Design review of the part built by this model. Coordinates are the model's own, in mm. Round coordinates to 2 decimals unless told otherwise and drop trailing zeros. Write each loop counter-clockwise with the first axis right and the second up, starting at its lowest first coordinate (ties: lowest second). Pieces come first, ordered by that corner, then holes. Notation, with made-up numbers: (-17.5, 80.5) -> (36.5, 80.5) arc R14 ccw to (36.5, 92.5) -> close; hole circle Ø5 at (56, -18.75). An arc over 180 degrees is marked (long way). One line per question, with ' | ' between items. Start each with the question number.
1) For probe 1 along Y at (x, z) = (0, 180.5); probe 2 along Y at (x, z) = (-195.5, -178.5); probe 3 along Z at (x, y) = (-315, -523.5), list the stretches that pass through material, from the lowest coordinate up.
2) Insertion check: pin 1 Ø1.2 at (x, z) = (-552, 936) entering from -Y; pin 2 Ø0.8 at (x, z) = (635, 935.5) entering from +Y; pin 3 Ø0.5 at (y, z) = (11.5, 935.5) entering from -X. Each pin has a flat end and moves straight along its axis. Give the tip position at first contact, or say it passes through.
3) Consider section A-A (z = 16). Give the boundary of the cut face in (x, y), then the cut area to 3 significant figures.
4) Consider section B-B (z = 795.5). Give the boundary of the cut face in (x, y).
```python
from build123d import *

# Parameters (mm, degrees)
SKETCH1_R           = 100
SKETCH1_R_2         = 45
BOSS_EXTRUDE1_DEPTH = 200
FILLET1_R           = 8
FILLET2_R           = 20
CUT_EXTRUDE1_DEPTH  = 200
SKETCH3_W           = 21.544123994
SKETCH3_H           = 11.057339859
BOSS_EXTRUDE2_DEPTH = 3
FILLET3_R           = 1.5
SKETCH4_R           = 1.289060933
SKETCH4_W           = 15.13149362
SKETCH4_H           = 3.065252971
SKETCH4_W_2         = 2.299952362
SKETCH4_H_2         = 2.429436964
SKETCH4_W_3         = 1.819095979
SKETCH4_H_3         = 1.788232519
SKETCH4_W_4         = 1.827971019
SKETCH4_W_5         = 1.693323788
SKETCH4_W_6         = 1.708755518
SKETCH4_W_7         = 1.86770952
SKETCH4_W_8         = 4.247138883
SKETCH4_W_9         = 4.75974501
SKETCH4_H_4         = 1.629278517
BOSS_EXTRUDE3_DEPTH = 0.2
SKETCH5_R           = 100
BOSS_EXTRUDE4_DEPTH = 8
SCALE1_SCALE        = 15.6
SCALE2_SCALE        = 0.5


with BuildPart() as part:
    # Sketch1 → Boss-Extrude1 (new body)
    with BuildSketch(Plane.XY):
        Circle(SKETCH1_R)
        Circle(SKETCH1_R_2, mode=Mode.SUBTRACT)
    extrude(amount=BOSS_EXTRUDE1_DEPTH)

    # Fillet1
    fillet1_edges = [part.edges().sort_by_distance(p)[0] for p in [
        (-100, 0, 200),
    ]]
    fillet(fillet1_edges, radius=FILLET1_R)

    # Fillet2
    fillet2_edges = [part.edges().sort_by_distance(p)[0] for p in [
        (-45, 0, 200),
    ]]
    fillet(fillet2_edges, radius=FILLET2_R)

    # Sketch2 → Cut-Extrude1 (cut)
    with BuildSketch(Plane(origin=(0, 0, 0), x_dir=(-1, 0, 0), z_dir=(0, 0, -1))):
        with BuildLine():
            Line((-28.43159427, -34.880430721), (28.43159427, -34.880430721))
            Line((28.43159427, -34.880430721), (28.43159427, -39.361060603))
            Line((28.43159427, -39.361060603), (11.44568617, -39.361060603))
            Line((11.44568617, -39.361060603), (11.44568617, -48.0006973))
            ThreePointArc((11.44568617, -48.0006973), (0, -49.480629882), (-11.44568617, -48.0006973))
            Line((-11.44568617, -48.0006973), (-11.44568617, -39.361060603))
            Line((-11.44568617, -39.361060603), (-28.43159427, -39.361060603))
            Line((-28.43159427, -39.361060603), (-28.43159427, -34.880430721))
        make_face()
    extrude(amount=-CUT_EXTRUDE1_DEPTH, mode=Mode.SUBTRACT)

    # Sketch3 → Boss-Extrude2 (add)
    with BuildSketch(Plane.XY.offset(200)):
        with Locations((78.121999913, 5.52866993)):
            Rectangle(SKETCH3_W, SKETCH3_H)
        with Locations((-78.121999913, 5.52866993)):
            Rectangle(SKETCH3_W, SKETCH3_H)
    extrude(amount=BOSS_EXTRUDE2_DEPTH)

    # Fillet3
    fillet3_edges = [part.edges().sort_by_distance(p)[0] for p in [
        (67.349937916, 11.057339859, 201.5),
        (67.349937916, 0, 201.5),
        (88.89406191, 0, 201.5),
        (88.89406191, 11.057339859, 201.5),
        (-88.89406191, 0, 201.5),
        (-67.349937916, 0, 201.5),
        (-67.349937916, 11.057339859, 201.5),
        (-88.89406191, 11.057339859, 201.5),
    ]]
    fillet(fillet3_edges, radius=FILLET3_R)

    # Sketch4 → Boss-Extrude3 (add)
    with BuildSketch(Plane.XY.offset(203)):
        with Locations((85.270492468, 1.703597588)):
            Circle(SKETCH4_R)
        with Locations((-85.270492468, 1.703597588)):
            Circle(SKETCH4_R)
        with Locations((76.415684726, 8.024713374)):
            Rectangle(SKETCH4_W, SKETCH4_H)
        with Locations((86.244085729, 8.342621377)):
            Rectangle(SKETCH4_W_2, SKETCH4_H_2)
        with Locations((69.759485906, 4.564769617)):
            Rectangle(SKETCH4_W_3, SKETCH4_H_3)
        with Locations((72.695697416, 4.564769617)):
            Rectangle(SKETCH4_W_4, SKETCH4_H_3)
        with Locations((75.569022832, 4.564769617)):
            Rectangle(SKETCH4_W_5, SKETCH4_H_3)
        with Locations((78.358433726, 4.564769617)):
            Rectangle(SKETCH4_W_6, SKETCH4_H_3)
        with Locations((81.259344257, 4.564769617)):
            Rectangle(SKETCH4_W_7, SKETCH4_H_3)
        with Locations((85.270492469, 4.564769617)):
            Rectangle(SKETCH4_W_8, SKETCH4_H_3)
        with Locations((71.229810421, 1.703597588)):
            Rectangle(SKETCH4_W_9, SKETCH4_H_4)
        with Locations((75.569022832, 1.703597588)):
            Rectangle(SKETCH4_W_5, SKETCH4_H_4)
        with Locations((78.358433726, 1.703597588)):
            Rectangle(SKETCH4_W_6, SKETCH4_H_4)
        with Locations((81.259344257, 1.703597588)):
            Rectangle(SKETCH4_W_7, SKETCH4_H_4)
        with Locations((-81.259344257, 1.703597588)):
            Rectangle(SKETCH4_W_7, SKETCH4_H_4)
        with Locations((-78.358433726, 1.703597588)):
            Rectangle(SKETCH4_W_6, SKETCH4_H_4)
        with Locations((-75.569022832, 1.703597588)):
            Rectangle(SKETCH4_W_5, SKETCH4_H_4)
        with Locations((-71.229810421, 1.703597588)):
            Rectangle(SKETCH4_W_9, SKETCH4_H_4)
        with Locations((-85.270492469, 4.564769617)):
            Rectangle(SKETCH4_W_8, SKETCH4_H_3)
        with Locations((-81.259344257, 4.564769617)):
            Rectangle(SKETCH4_W_7, SKETCH4_H_3)
        with Locations((-78.358433726, 4.564769617)):
            Rectangle(SKETCH4_W_6, SKETCH4_H_3)
        with Locations((-75.569022832, 4.564769617)):
            Rectangle(SKETCH4_W_5, SKETCH4_H_3)
        with Locations((-72.695697416, 4.564769617)):
            Rectangle(SKETCH4_W_4, SKETCH4_H_3)
        with Locations((-69.759485906, 4.564769617)):
            Rectangle(SKETCH4_W_3, SKETCH4_H_3)
        with Locations((-86.244085729, 8.342621377)):
            Rectangle(SKETCH4_W_2, SKETCH4_H_2)
        with Locations((-76.415684726, 8.024713374)):
            Rectangle(SKETCH4_W, SKETCH4_H)
    extrude(amount=BOSS_EXTRUDE3_DEPTH)

    # Sketch5 → Boss-Extrude4 (add)
    with BuildSketch(Plane(origin=(0, 0, 0), x_dir=(-1, 0, 0), z_dir=(0, 0, -1))):
        Circle(SKETCH5_R)
        with BuildLine():
            Line((-28.43159427, -39.361060603), (-28.43159427, -34.880430721))
            ThreePointArc((-28.43159427, -34.880430721), (0, 45), (28.43159427, -34.880430721))
            Line((28.43159427, -34.880430721), (28.43159427, -39.361060603))
            Line((28.43159427, -39.361060603), (21.810706275, -39.361060603))
            ThreePointArc((21.810706275, -39.361060603), (16.757721923, -41.763366195), (11.44568617, -43.520067418))
            Line((11.44568617, -43.520067418), (11.44568617, -45.760382359))
            Line((11.44568617, -45.760382359), (11.44568617, -48.0006973))
            ThreePointArc((11.44568617, -48.0006973), (0, -49.480629882), (-11.44568617, -48.0006973))
            Line((-11.44568617, -48.0006973), (-11.44568617, -43.520067418))
            ThreePointArc((-11.44568617, -43.520067418), (-16.757721923, -41.763366195), (-21.810706275, -39.361060603))
            Line((-21.810706275, -39.361060603), (-28.43159427, -39.361060603))
        make_face(mode=Mode.SUBTRACT)
    extrude(amount=BOSS_EXTRUDE4_DEPTH)


with BuildPart() as part_1:
    # Scale1: scaled about (-1e-09, 0.224288637, 95.374877124)
    add(part.part.scale(SCALE1_SCALE).moved(Location((1.5e-08, -3.2746141, -1392.47320601))))


with BuildPart() as part_2:
    # Scale2: scaled about (-5e-09, 0.224288632, 95.374877131)
    add(part_1.part.scale(SCALE2_SCALE).moved(Location((-3e-09, 0.112144316, 47.687438566))))


solid = part_2.part
```
From the geometry:
1) probe 1: y = -781.53 to -387.47, 349.47 to 778.47 | probe 2: y = -756.63 to -308.54, 289.99 to 753.58 | probe 3: z = -710.95 to 911.45
2) pin 1: stops at y = 5.41 | pin 2: stops at y = 73.02 | pin 3: stops at x = -675.16
3) outline: circle Ø1560 at (0, -1.53); hole (-221.77, -308.54) -> (-170.12, -308.54) arc R351 ccw to (-89.28, -340.98) -> (-89.28, -375.93) arc R351 ccw to (89.28, -375.93) -> (89.28, -340.98) arc R351 ccw to (170.12, -308.54) -> (221.77, -308.54) -> (221.77, -273.59) arc R351 ccw (long way) to (-221.77, -273.59) -> close | area: 1,520,000 mm2
4) outline: circle Ø1560 at (0, -1.53); hole (-221.77, -308.54) -> (-180.66, -308.54) arc R356.23 ccw to (-89.28, -346.39) -> (-89.28, -375.93) arc R351 ccw to (89.28, -375.93) -> (89.28, -346.39) arc R356.23 ccw to (180.66, -308.54) -> (221.77, -308.54) -> (221.77, -280.31) arc R356.23 ccw (long way) to (-221.77, -280.31) -> close
